from build123d import *

# Parameters (mm, degrees)
F0_W     = 200
F0_H     = 145
F0_W_2   = 3
F0_H_2   = 5
F0_R     = 1.5
F0_W_3   = 5
F0_H_3   = 3
F0_W_4   = 10
F0_R_2   = 2
F0_H_4   = 10
F0_R_3   = 3.25
F0_R_4   = 10
F0_H_5   = 135
F1_DEPTH = 3


with BuildPart() as f1:
    # F0 (on Top) → F1 (new body)
    with BuildSketch(Plane.XY):
        with Locations((6.405575, -4.149114)):
            Rectangle(F0_W, F0_H)
        with Locations((-79.344425, -71.149114)):
            Rectangle(F0_W_2, F0_H_2, mode=Mode.SUBTRACT)
        with Locations((-79.344425, -64.149114)):
            Circle(F0_R, mode=Mode.SUBTRACT)
        with Locations((-69.344425, -64.149114)):
            Rectangle(F0_W_3, F0_H_3, mode=Mode.SUBTRACT)
        with Locations((-52.594425, -71.649114)):
            Rectangle(F0_W_4, F0_H_3, mode=Mode.SUBTRACT)
        with Locations((-79.344425, -57.149114)):
            Rectangle(F0_W_2, F0_H_2, mode=Mode.SUBTRACT)
        with Locations((-41.094425, -71.649114)):
            Circle(F0_R, mode=Mode.SUBTRACT)
        with Locations((-29.594425, -71.649114)):
            Rectangle(F0_W_4, F0_H_3, mode=Mode.SUBTRACT)
        with Locations((-79.344425, -34.149114)):
            Circle(F0_R_2, mode=Mode.SUBTRACT)
        with Locations((-88.596009, -15.649114)):
            Rectangle(F0_W_2, F0_H_4, mode=Mode.SUBTRACT)
        with Locations((-81.594425, -9.149114)):
            Circle(F0_R, mode=Mode.SUBTRACT)
        with Locations((-22.594425, -14.149114)):
            Circle(F0_R_2, mode=Mode.SUBTRACT)
        with Locations((-34.594425, -9.149114)):
            Circle(F0_R, mode=Mode.SUBTRACT)
        with Locations((42.405575, -71.649114)):
            Rectangle(F0_W_4, F0_H_3, mode=Mode.SUBTRACT)
        with Locations((53.905575, -71.649114)):
            Circle(F0_R, mode=Mode.SUBTRACT)
        with Locations((54.905575, -64.149114)):
            Circle(F0_R_3, mode=Mode.SUBTRACT)
        with Locations((65.405575, -71.649114)):
            Rectangle(F0_W_4, F0_H_3, mode=Mode.SUBTRACT)
        with Locations((93.405575, -64.149114)):
            Circle(F0_R_3, mode=Mode.SUBTRACT)
        with Locations((54.905575, -25.649114)):
            Circle(F0_R_3, mode=Mode.SUBTRACT)
        with Locations((32.405575, -6.649114)):
            Rectangle(F0_W_4, F0_H_3, mode=Mode.SUBTRACT)
        with Locations((43.905575, -6.649114)):
            Circle(F0_R, mode=Mode.SUBTRACT)
        with Locations((55.405575, -6.649114)):
            Rectangle(F0_W_4, F0_H_3, mode=Mode.SUBTRACT)
        with Locations((93.405575, -25.649114)):
            Circle(F0_R_3, mode=Mode.SUBTRACT)
        with Locations((-88.594425, -4.149114)):
            Circle(F0_R, mode=Mode.SUBTRACT)
        with Locations((-81.594425, 0.850886)):
            Circle(F0_R, mode=Mode.SUBTRACT)
        with Locations((-68.594425, -4.149114)):
            Circle(F0_R_4, mode=Mode.SUBTRACT)
        with Locations((-88.596009, 7.350886)):
            Rectangle(F0_W_2, F0_H_4, mode=Mode.SUBTRACT)
        with Locations((-79.344425, 25.850886)):
            Circle(F0_R_2, mode=Mode.SUBTRACT)
        with Locations((-34.594425, 0.850886)):
            Circle(F0_R, mode=Mode.SUBTRACT)
        with Locations((-22.594425, -4.149114)):
            Circle(F0_R_2, mode=Mode.SUBTRACT)
        with Locations((-22.594425, 5.850886)):
            Circle(F0_R_2, mode=Mode.SUBTRACT)
        with Locations((-13.596009, 16.850886)):
            Rectangle(F0_W_2, F0_H_4, mode=Mode.SUBTRACT)
        with Locations((-13.594425, 28.350886)):
            Circle(F0_R, mode=Mode.SUBTRACT)
        with Locations((-79.344425, 48.850886)):
            Rectangle(F0_W_2, F0_H_2, mode=Mode.SUBTRACT)
        with Locations((-79.344425, 55.850886)):
            Circle(F0_R, mode=Mode.SUBTRACT)
        with Locations((-69.344425, 55.850886)):
            Rectangle(F0_W_3, F0_H_3, mode=Mode.SUBTRACT)
        with Locations((-79.344425, 62.850886)):
            Rectangle(F0_W_2, F0_H_2, mode=Mode.SUBTRACT)
        with Locations((-52.594425, 63.350886)):
            Rectangle(F0_W_4, F0_H_3, mode=Mode.SUBTRACT)
        with Locations((-13.596009, 39.850886)):
            Rectangle(F0_W_2, F0_H_4, mode=Mode.SUBTRACT)
        with Locations((-41.094425, 63.350886)):
            Circle(F0_R, mode=Mode.SUBTRACT)
        with Locations((-29.594425, 63.350886)):
            Rectangle(F0_W_4, F0_H_3, mode=Mode.SUBTRACT)
        with Locations((54.905575, 17.350886)):
            Circle(F0_R_3, mode=Mode.SUBTRACT)
        with Locations((101.405575, -4.149114)):
            Rectangle(F0_W_2, F0_H_5, mode=Mode.SUBTRACT)
        with Locations((93.405575, 17.350886)):
            Circle(F0_R_3, mode=Mode.SUBTRACT)
        with Locations((54.905575, 55.850886)):
            Circle(F0_R_3, mode=Mode.SUBTRACT)
        with Locations((42.405575, 63.350886)):
            Rectangle(F0_W_4, F0_H_3, mode=Mode.SUBTRACT)
        with Locations((53.905575, 63.350886)):
            Circle(F0_R, mode=Mode.SUBTRACT)
        with Locations((65.405575, 63.350886)):
            Rectangle(F0_W_4, F0_H_3, mode=Mode.SUBTRACT)
        with Locations((93.405575, 55.850886)):
            Circle(F0_R_3, mode=Mode.SUBTRACT)
    extrude(amount=F1_DEPTH)


solid = f1.part
Verification items for the finished model (mm, model axes). Give positions to 0.01 mm unless a question says otherwise; leave off trailing zeros. Order: outer loops, then holes, each group sorted by start corner. A loop starts at its lowest first (then second) coordinate and runs counter-clockwise, first axis right, second up. Notation, with made-up numbers: M 57,61.25 L 113,61.25 A9 ccw 113,71.25 Z; hole C -40,45.25 d6. An arc over 180 degrees is marked long. Answer as a JSON object with one key per item and string values. Group by question number.
1) Depth check by flat-ended pin: pin 1 Ø6 at (x, y) = (54.91, -25.65) entering from -Z. Enter the tip coordinate at first touch or a pass-through.
2) Cross-section at A-A (x = -53.5). Enter the section's corners in (y, z).
3) Mould release check, pull along X, two halves, no side actions. Record for faces 1 (the face through (5, -3, 3)), 2 (the face through (96.505, -24.673, 1.479)): released by +X, released by -X, zero draft, split by the parting line, or undercut.
4) Scan lines: line 1 along Y through (x, z) = (-26, 0.4); line 2 along X through (y, z) = (61, 1.75); line 3 along Y through (x, z) = (51, 1.75). Record each from-to range of solid material in increasing order. Write a range as [from, to].
5) Cross-section at B-B (z = 2.4). Give the number of separate pieces and of enclosed holes in the cut face, then the cut area to 3 significant figures.
Result sheet:
{
 "1": {"pin 1": "passes through"},
 "2": {"outline": "M -76.65,0 L -73.15,0 L -73.15,3 L -76.65,3 Z; M -70.15,0 L 61.85,0 L 61.85,3 L -70.15,3 Z; M 64.85,0 L 68.35,0 L 68.35,3 L 64.85,3 Z"},
 "3": {"face 1": "zero draft", "face 2": "undercut"},
 "4": {"line 1": "y = [-76.65, -73.15], [-70.15, 61.85], [64.85, 68.35]", "line 2": "x = [-93.59, -80.84], [-77.84, 99.91], [102.91, 106.41]", "line 3": "y = [-76.65, -8.15], [-5.15, 68.35]"},
 "5": {"separate pieces": "1", "enclosed holes": "48", "area": "27,400 mm2"}
}
